from build123d import *

# Parameters (mm, degrees)
SKETCH_1_R          = 2
EXTRUDE_1_DEPTH     = 60
CUT_EXTRUDE_1_DEPTH = 55


with BuildPart() as part:
    # 草图1 → 凸台-拉伸1 (new body)
    with BuildSketch(Plane.XY):
        with BuildLine():
            Line((10.155709238, 10.284373102), (10.155709238, 14.620809902))
            add(Edge.make_bspline(
                [(10.155709238, 14.620809902), (-1.633651532, 8.235919316), (-14.844290763, 10.284373103)],
                knots=[0, 0, 0, 1, 1, 1], degree=2))
            Line((-14.844290763, 10.284373103), (-14.844290762, -7.879190098))
            Line((-14.844290762, -7.879190098), (2.430284378, -13.492039805))
            add(Edge.make_bspline(
                [(2.430284378, -13.492039805), (4.564401085, -0.294968248), (14.279905714, 8.944340437)],
                knots=[0, 0, 0, 1, 1, 1], degree=2))
            Line((14.279905714, 8.944340437), (10.155709238, 10.284373102))
        make_face()
        with Locations((-3.844290762, 0.11277771)):
            Circle(SKETCH_1_R, mode=Mode.SUBTRACT)
        with Locations((3.155709238, 5.198575406)):
            Circle(SKETCH_1_R, mode=Mode.SUBTRACT)
    extrude(amount=EXTRUDE_1_DEPTH)

    # 草图2 → 切除-拉伸1 (cut)
    with BuildSketch(Plane(origin=(0, 0, 0), x_dir=(-1, 0, 0), z_dir=(0, 0, -1))):
        with BuildLine():
            Line((-0.804568229, 8.434643384), (6.195431771, 3.348845688))
            ThreePointArc((6.195431771, 3.348845688), (7.08035874, -2.238363299), (1.493149753, -3.123290267))
            Line((1.493149753, -3.123290267), (-5.506850247, 1.962507429))
            ThreePointArc((-5.506850247, 1.962507429), (-6.391777215, 7.549716416), (-0.804568229, 8.434643384))
        make_face()
    extrude(amount=-CUT_EXTRUDE_1_DEPTH, mode=Mode.SUBTRACT)


solid = part.part
Read the model definition and answer for the solid it produces. Units are mm, in the model's axes. A direction names the side the tool comes from. Coordinates: 2 decimals unless noted, no trailing zeros. Answer as a JSON object with one key per item and string values.
1) The mould has two halves that part along Y. Classify faces 1 (the face through (-7.13, -2.17, 27.12)), 2 (the face through (12.247, 9.605, 29.58)), 3 (the face through (0, 1, 60)), 4 (the face through (-6.328, -10.646, 29.58)): released by +Y, released by -Y, zero draft, split by the parting line, or undercut.
Model answer:
{"face 1": "undercut", "face 2": "released by +Y", "face 3": "zero draft", "face 4": "released by -Y"}
2) Consider line 1 along X through (y, z) = (3.75, 14.5); line 2 along Y through (x, z) = (-2, 40); line 3 along Y through (x, z) = (5, 3). Determine where each line is inside the solid, lowest interval first. Write a range as from..to.
Model answer:
{"line 1": "x = -14.84..-5.64, 6.88..9.65", "line 2": "y = -12.05..-3.44, 6.4..10.34", "line 3": "y = -4.38..1.59, 8.75..12.26"}
3) A cutting plane is placed at A-A, the plane z = 56. State how many separate pieces and enclosed holes the cut face has, plus the area to 3 significant figures.
Model answer:
{"separate pieces": "1", "enclosed holes": "2", "area": "465 mm²"}
4) A tool of negligible diameter and unlimited length cuts with its end or side. For faces 5 (the face through (-2.646, 5.927, 27.115)), 6 (the face through (10.156, 12, 30)), 7 (the face through (-1.937, 0.714, 57.465)), from which of +Z, -Z, +X, -X, +Y, -Y can it reach the whole face along a straight path? Write none if from no direction.
Model answer:
{"face 5": "-Z", "face 6": "+Z, -Z, +X, +Y", "face 7": "+Z, -Z"}
5) Each of these flat-tipped pins is pushed along its axis until it touches: pin 1 (12 mm diameter, centred on x = -8, z = 52.5, fed in from -Y); pin 2 (5 mm diameter, centred on x = -10.5, z = 41, fed in from +Y); pin 3 (1 mm diameter, centred on x = -6, z = 41, fed in from +Y). Where does it stop, or does it pass through?
Model answer:
{"pin 1": "stops at y = -12.05", "pin 2": "stops at y = 10.04", "pin 3": "stops at y = 9.9"}
